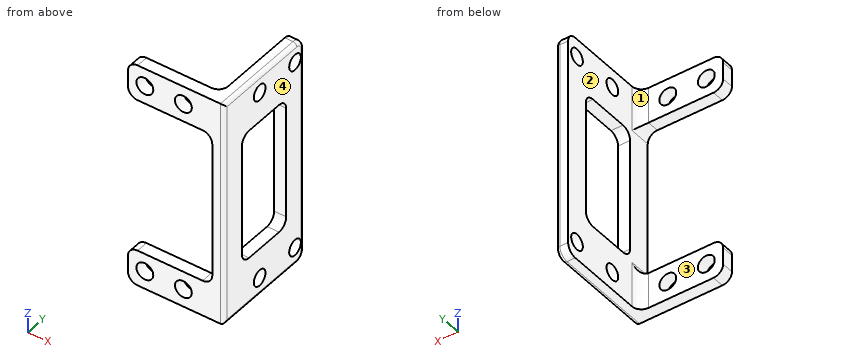
```python
from build123d import *

# Parameters (mm, degrees)
BOSS_EXTRUDE1_DEPTH = 3.175
SKETCH2_R           = 2.2225
CUT_EXTRUDE1_DEPTH  = 57.960207911
SKETCH5_W           = 3.175
SKETCH5_H           = 60.198
BOSS_EXTRUDE3_DEPTH = 25.4
SKETCH6_R           = 2.0955
CUT_EXTRUDE3_DEPTH  = 67.208578827
SKETCH8_W           = 34.798
SKETCH8_H           = 15.875
CUT_EXTRUDE4_DEPTH  = 67.208578827
FILLET1_R           = 2.54
FILLET2_R           = 1


with BuildPart() as part:
    # Sketch1 → Boss-Extrude1 (new body)
    with BuildSketch(Plane(origin=(0, 0, 0), x_dir=(1, 0, 0), z_dir=(0, 1, 0))):
        Polygon((-12.7, -4.7625), (-12.7, 4.7625), (12.7, 4.7625), (12.7, -4.7625), (12.7, -45.9105), (12.7, -55.4355), (-12.7, -55.4355), (-12.7, -45.9105), (9.525, -45.9105), (9.525, -4.7625), align=None)
    extrude(amount=BOSS_EXTRUDE1_DEPTH)

    # Sketch2 → Cut-Extrude1 (cut, through all)
    with BuildSketch(Plane(origin=(0, 3.175, 0), x_dir=(1, 0, 0), z_dir=(0, 1, 0))):
        with Locations(Location((-8.255, 0, 0), (0, 0, 270))):
            Circle(SKETCH2_R)
        with Locations(Location((1.905, 0, 0), (0, 0, 270))):
            Circle(SKETCH2_R)
        with Locations(Location((-8.255, -50.673, 0), (0, 0, 270))):
            Circle(SKETCH2_R)
        with Locations(Location((1.905, -50.673, 0), (0, 0, 270))):
            Circle(SKETCH2_R)
    extrude(amount=-CUT_EXTRUDE1_DEPTH, mode=Mode.SUBTRACT)

    # Sketch5 → Boss-Extrude3 (add)
    with BuildSketch(Plane(origin=(0, 3.175, 0), x_dir=(1, 0, 0), z_dir=(0, 1, 0))):
        with Locations((11.1125, -25.3365)):
            Rectangle(SKETCH5_W, SKETCH5_H)
    extrude(amount=BOSS_EXTRUDE3_DEPTH)

    # Sketch6 → Cut-Extrude3 (cut, through all)
    with BuildSketch(Plane.ZY.offset(-9.525)):
        with Locations((0, 25.4)):
            Circle(SKETCH6_R)
        with Locations((0, 12.7)):
            Circle(SKETCH6_R)
        with Locations((50.673, 25.4)):
            Circle(SKETCH6_R)
        with Locations((50.673, 12.7)):
            Circle(SKETCH6_R)
    extrude(amount=-CUT_EXTRUDE3_DEPTH, mode=Mode.SUBTRACT)

    # Sketch8 → Cut-Extrude4 (cut, through all)
    with BuildSketch(Plane.ZY.offset(-9.525)):
        with Locations((25.3365, 14.2875)):
            Rectangle(SKETCH8_W, SKETCH8_H)
    extrude(amount=-CUT_EXTRUDE4_DEPTH, mode=Mode.SUBTRACT)

    # Fillet1
    fillet1_edges = [part.edges().sort_by_distance(p)[0] for p in [
        (-12.7, 1.5875, 4.7625),
        (-12.7, 1.5875, -4.7625),
        (11.1125, 28.575, -4.7625),
        (11.1125, 28.575, 55.4355),
        (-12.7, 1.5875, 55.4355),
        (-12.7, 1.5875, 45.9105),
        (9.525, 1.5875, 45.9105),
        (9.525, 1.5875, 4.7625),
        (9.525, 3.175, 0),
        (9.525, 3.175, 50.673),
        (11.1125, 6.35, 42.7355),
        (11.1125, 22.225, 42.7355),
        (11.1125, 22.225, 7.9375),
        (11.1125, 6.35, 7.9375),
    ]]
    fillet(fillet1_edges, radius=FILLET1_R)

    # Fillet2
    fillet2_edges = [part.edges().sort_by_distance(p)[0] for p in [
        (12.7, 13.0175, -4.7625),
        (12.7, 28.575, 25.3365),
        (12.7, 13.0175, 55.4355),
        (12.7, 27.831051224, 54.691551224),
        (12.7, 27.831051224, -4.018551224),
        (12.7, 0, 25.3365),
    ]]
    fillet(fillet2_edges, radius=FILLET2_R)


solid = part.part
```
Geometry check sheet. Reference: the model listing, model coordinates, mm. Face numbers are marked on the shaded views. A direction names the side the tool comes from. Coordinates: 2 decimals unless noted, no trailing zeros. Order: outer loops, then holes, each group sorted by start corner. A loop starts at its lowest first (then second) coordinate and runs counter-clockwise, first axis right, second up. Notation, with made-up numbers: (6.25, 75.5) - (19.25, 75.5) arc R20 cw to (19.25, 106.5) - close; hole circle Ø8 at (-33, 42.5). An arc over 180 degrees is marked (long way). Answer as a JSON object with one key per item and string values. Group by question number.
Item 1: Scan lines: probe 1 along Y at (x, z) = (11.2, 0) (1 decimal); probe 2 along Z at (x, y) = (11.5, 11.5); probe 3 along X at (y, z) = (4.75, 35.5) (3 decimals). Record each from-to range of solid material in increasing order.
Item 2: Draft check along Z on the marked faces 1 and 2. Enter one of: +Z half, -Z half, draft (parallel to the pull), parting line (faces both ways), or undercut.
Item 3: Sectioned sample at B-B, the plane z = 18.5. Record the cut outline in (x, y) (3 decimals), and give its area (3 significant figures).
Item 4: Tool access check on the marked faces 3 and 4. Record the directions out of +Z, -Z, +X, -X, +Y, -Y that give a thin tool (end or side, any length) a straight path to the whole face; none if there is none.
Item 5: Sectioned sample at C-C, the plane y = 12.7. Record the cut outline in (x, z) (1 decimal).
Item 6: Depth check by flat-ended pin: pin 1 Ø6 at (x, z) = (1.905, 0) entering from +Y (3 decimals); pin 2 Ø14.5 at (y, z) = (18, 25) entering from -X (3 decimals); pin 3 Ø4 at (y, z) = (4.5, 46.5) entering from -X. Enter the tip coordinate at first touch or a pass-through.
Item 7: Sectioned sample at A-A, the plane x = -4. Record the cut outline in (y, z) (1 decimal).
Item 8: Sectioned sample at D-D, the plane x = 10.5. Give the number of separate pieces and of enclosed holes in the cut face, and give its area (3 significant figures).
Resolved:
{
 "1": {"probe 1": "0 to 10.6, 14.8 to 23.3, 27.5 to 28.6", "probe 2": "-4.76 to -1.72, 1.72 to 7.94, 42.74 to 48.96, 52.39 to 55.44", "probe 3": "9.525 to 12.7"},
 "2": {"face 1": "draft", "face 2": "undercut"},
 "3": {"outline": "(9.525, 0) - (11.7, 0) arc R1 ccw to (12.7, 1) - (12.7, 6.35) - (9.525, 6.35) - close; (9.525, 22.225) - (12.7, 22.225) - (12.7, 27.575) arc R1 ccw to (11.7, 28.575) - (9.525, 28.575) - close", "area": "39.9 mm^2"},
 "4": {"face 3": "+Z, -Z, -X, +Y", "face 4": "+Z, -Z, +X, +Y, -Y"},
 "5": {"outline": "(9.5, -4.8) - (11.7, -4.8) arc R1 ccw to (12.7, -3.8) - (12.7, -2.1) - (9.5, -2.1) - close; (9.5, 2.1) - (12.7, 2.1) - (12.7, 7.9) - (9.5, 7.9) - close; (9.5, 42.7) - (12.7, 42.7) - (12.7, 48.6) - (9.5, 48.6) - close; (9.5, 52.8) - (12.7, 52.8) - (12.7, 54.4) arc R1 ccw to (11.7, 55.4) - (9.5, 55.4) - close"},
 "6": {"pin 1": "y = 3.175", "pin 2": "x = 9.525", "pin 3": "x = -12.66"},
 "7": {"outline": "(0, -4.8) - (3.2, -4.8) - (3.2, 4.8) - (0, 4.8) - close; (0, 45.9) - (3.2, 45.9) - (3.2, 55.4) - (0, 55.4) - close"},
 "8": {"separate pieces": "1", "enclosed holes": "5", "area": "1,120 mm^2"}
}
